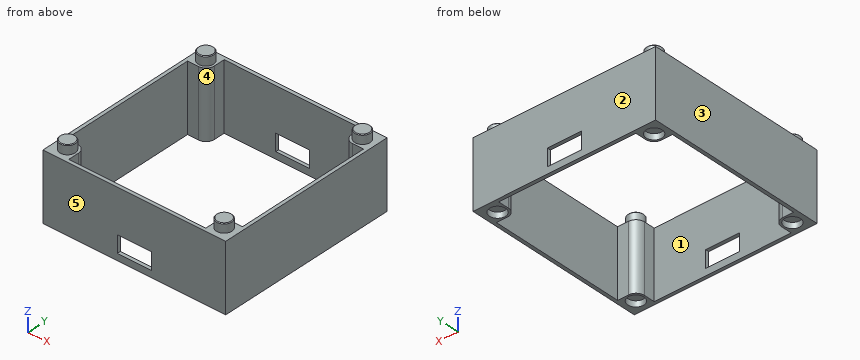
from build123d import *

# Parameters (mm, degrees)
SKICA1_W                 = 5.8
SKICA1_H                 = 5.8
SKICA1_W_2               = 1
SKICA1_H_2               = 41
SKICA1_W_3               = 41
SKICA1_H_3               = 1
P_IDAT_VYSUNUT_M2_DEPTH  = 20
ZAOBLIT1_R               = 2.5
SKICA2_R                 = 2.4
ODEBRAT_VYSUNUT_M1_DEPTH = 1.7
SKICA3_R                 = 2.3
P_IDAT_VYSUNUT_M3_DEPTH  = 2.7
ZKOSEN_1_SIZE            = 0.2
SKICA4_W                 = 10.16
SKICA4_H                 = 5.08
ODEBRAT_VYSUNUT_M2_DEPTH = 68.7


with BuildPart() as part:
    # Skica1 → Přidat vysunutím2 (new body)
    with BuildSketch(Plane.XY):
        Polygon((-27.3, 27.3), (-27.3, 20.5), (-26.3, 20.5), (-26.3, 26.3), (-20.5, 26.3), (-20.5, 27.3), align=None)
        with Locations((-23.4, 23.4)):
            Rectangle(SKICA1_W, SKICA1_H)
        Polygon((26.3, 20.5), (27.3, 20.5), (27.3, 27.3), (20.5, 27.3), (20.5, 26.3), (26.3, 26.3), align=None)
        with Locations((23.4, 23.4)):
            Rectangle(SKICA1_W, SKICA1_H)
        Polygon((20.5, -26.3), (20.5, -27.3), (27.3, -27.3), (27.3, -20.5), (26.3, -20.5), (26.3, -26.3), align=None)
        with Locations((23.4, -23.4)):
            Rectangle(SKICA1_W, SKICA1_H)
        with Locations((-23.4, -23.4)):
            Rectangle(SKICA1_W, SKICA1_H)
        Polygon((-27.3, -27.3), (-20.5, -27.3), (-20.5, -26.3), (-26.3, -26.3), (-26.3, -20.5), (-27.3, -20.5), align=None)
        with Locations((-26.8, 0)):
            Rectangle(SKICA1_W_2, SKICA1_H_2)
        with Locations((0, -26.8)):
            Rectangle(SKICA1_W_3, SKICA1_H_3)
        with Locations((26.8, 0)):
            Rectangle(SKICA1_W_2, SKICA1_H_2)
        with Locations((0, 26.8)):
            Rectangle(SKICA1_W_3, SKICA1_H_3)
    extrude(amount=P_IDAT_VYSUNUT_M2_DEPTH)

    # Zaoblit1
    zaoblit1_edges = [part.edges().sort_by_distance(p)[0] for p in [
        (20.5, -20.5, 10),
        (20.5, 20.5, 10),
        (-20.5, 20.5, 10),
        (-20.5, -20.5, 10),
    ]]
    fillet(zaoblit1_edges, radius=ZAOBLIT1_R)

    # Skica2 → Odebrat vysunutím1 (cut)
    with BuildSketch(Plane(origin=(0, 0, 0), x_dir=(-1, 0, 0), z_dir=(0, 0, -1))):
        with Locations((-23.4, 23.4)):
            Circle(SKICA2_R)
        with Locations((23.4, 23.4)):
            Circle(SKICA2_R)
        with Locations((23.4, -23.4)):
            Circle(SKICA2_R)
        with Locations((-23.4, -23.4)):
            Circle(SKICA2_R)
    extrude(amount=-ODEBRAT_VYSUNUT_M1_DEPTH, mode=Mode.SUBTRACT)

    # Skica3 → Přidat vysunutím3 (add)
    with BuildSketch(Plane.XY.offset(20)):
        with Locations((-23.4, 23.4)):
            Circle(SKICA3_R)
        with Locations((23.4, 23.4)):
            Circle(SKICA3_R)
        with Locations((23.4, -23.4)):
            Circle(SKICA3_R)
        with Locations((-23.4, -23.4)):
            Circle(SKICA3_R)
    extrude(amount=P_IDAT_VYSUNUT_M3_DEPTH)

    # Zkosení1
    zkosen_1_edges = [part.edges().sort_by_distance(p)[0] for p in [
        (-25.7, 23.4, 22.7),
        (21.1, 23.4, 22.7),
        (21.1, -23.4, 22.7),
        (-25.7, -23.4, 22.7),
    ]]
    chamfer(zkosen_1_edges, length=ZKOSEN_1_SIZE)

    # Skica4 → Odebrat vysunutím2 (cut)
    with BuildSketch(Plane(origin=(0, -27.3, 0), x_dir=(-1, 0, 0), z_dir=(0, -1, 0))):
        with Locations((0, -4.54)):
            Rectangle(SKICA4_W, SKICA4_H)
    extrude(amount=-ODEBRAT_VYSUNUT_M2_DEPTH, mode=Mode.SUBTRACT)


solid = part.part
Geometry: final body of the model. Coordinates: model frame, mm. Face numbers are marked on the shaded views. A direction names the side the tool comes from. Coordinates: 2 decimals unless noted, no trailing zeros. Order: outer loops, then holes, each group sorted by start corner. A loop starts at its lowest first (then second) coordinate and runs counter-clockwise, first axis right, second up.
(1) Section query B-B (x = -8.5). Return the cut outline in (y, z).
(2) First-contact query: pin 1 (0.5 mm diameter, centred on x = 1.5, y = 27, fed in from +Z); pin 2 (3 mm diameter, centred on x = -23.4, y = -23.4, fed in from -Z). Flat tips, straight axial feed; report the tip coordinate or a pass-through.
(3) Section query A-A (z = 4.25). Return the cut outline in (x, y).
(4) Draft query along Y for the marked faces 3, 4 and 5. Return one class per face: pulls with the +Y half, pulls with the -Y half, needs draft (parallel to the pull), parting line crosses it, or undercut.
(5) Material intervals for probe 1 along X at (y, z) = (-3, 7.75); probe 2 along X at (y, z) = (23, 1.75), sorted ascending.
(6) Section query D-D (z = 8.75). Return the cut outline in (x, y), plus the area to 3 significant figures.
(7) Access query for the marked faces 1 and 2. Directions: +Z, -Z, +X, -X, +Y, -Y. A direction counts if a zero-diameter tool reaches every point of the face in a straight line with its end or side. Return the directions, or none.
Solution:
1. outline: (-27.3, 0) - (-26.3, 0) - (-26.3, 20) - (-27.3, 20) - close; (26.3, 0) - (27.3, 0) - (27.3, 20) - (26.3, 20) - close
2. pin 1: stops at z = 20
2. pin 2: stops at z = 1.7
3. outline: (-27.3, -27.3) - (-5.08, -27.3) - (-5.08, -26.3) - (-20.5, -26.3) - (-20.5, -23) arc R2.5 ccw to (-23, -20.5) - (-26.3, -20.5) - (-26.3, 20.5) - (-23, 20.5) arc R2.5 ccw to (-20.5, 23) - (-20.5, 26.3) - (-5.08, 26.3) - (-5.08, 27.3) - (-27.3, 27.3) - close; (5.08, -27.3) - (27.3, -27.3) - (27.3, 27.3) - (5.08, 27.3) - (5.08, 26.3) - (20.5, 26.3) - (20.5, 23) arc R2.5 ccw to (23, 20.5) - (26.3, 20.5) - (26.3, -20.5) - (23, -20.5) arc R2.5 ccw to (20.5, -23) - (20.5, -26.3) - (5.08, -26.3) - close
4. face 3: needs draft
4. face 4: undercut
4. face 5: pulls with the -Y half
5. probe 1: x = -27.3 to -26.3, 26.3 to 27.3
5. probe 2: x = -27.3 to -20.5, 20.5 to 27.3
6. outline: (-27.3, -27.3) - (27.3, -27.3) - (27.3, 27.3) - (-27.3, 27.3) - close; hole (-26.3, -20.5) - (-23, -20.5) arc R2.5 cw to (-20.5, -23) - (-20.5, -26.3) - (20.5, -26.3) - (20.5, -23) arc R2.5 cw to (23, -20.5) - (26.3, -20.5) - (26.3, 20.5) - (23, 20.5) arc R2.5 cw to (20.5, 23) - (20.5, 26.3) - (-20.5, 26.3) - (-20.5, 23) arc R2.5 cw to (-23, 20.5) - (-26.3, 20.5) - close
6. area: 344 mm2
7. face 1: +Z, -Z
7. face 2: +Z, -Z, +X, -X, +Y
